Part model, mm, in its own coordinate system. A direction names the side the tool comes from. Coordinates: 2 decimals unless noted, no trailing zeros. Order: outer loops, then holes, each group sorted by start corner. A loop starts at its lowest first (then second) coordinate and runs counter-clockwise, first axis right, second up. Notation, with made-up numbers: M 62.5,63.25 L 120.5,63.25 A25 cw 120.5,96.25 Z; hole C -12,3.25 d4. An arc over 180 degrees is marked long. Answer in a Markdown table with one row per item. Add a question column.
from build123d import *

# Parameters (mm, degrees)
SKETCH1_W             = 24
SKETCH1_H             = 40
BOSS_EXTRUDE1_DEPTH   = 10
SKETCH2_R             = 4
BOSS_EXTRUDE2_DEPTH   = 10
SKETCH4_W             = 2
SKETCH4_H             = 15
CUT_EXTRUDE1_DEPTH    = 20
SKETCH5_R             = 2.4
CUT_EXTRUDE2_DEPTH    = 56
CHAMFER2_SIZE         = 2
CHAMFER3_SIZE2        = 2
CHAMFER3_SIZE         = 5.63516655
CHAMFER3_EDGE_2_SIZE2 = 5.63516655
CHAMFER3_EDGE_2_SIZE  = 2
CHAMFER3_EDGE_3_SIZE2 = 2
CHAMFER3_EDGE_3_SIZE  = 5.63516655
CHAMFER3_EDGE_4_SIZE2 = 5.63516655
CHAMFER3_EDGE_4_SIZE  = 2
FILLET2_R             = 3


with BuildPart() as part:
    # Sketch1 → Boss-Extrude1 (new body)
    with BuildSketch(Plane(origin=(0, 0, 0), x_dir=(1, 0, 0), z_dir=(0, 1, 0))):
        Rectangle(SKETCH1_W, SKETCH1_H)
    extrude(amount=BOSS_EXTRUDE1_DEPTH)

    # Sketch2 → Boss-Extrude2 (add)
    with BuildSketch(Plane.XZ):
        Polygon((-12, -20), (-12, 30), (-27, 30), (-27, -20), (-10, -30), (-10, -45), (10, -45), (10, -30), (27, -20), (27, 30), (12, 30), (12, -20), align=None)
        with Locations((0, -34)):
            Circle(SKETCH2_R, mode=Mode.SUBTRACT)
        with Locations((-19.5, 19)):
            Circle(SKETCH2_R, mode=Mode.SUBTRACT)
        with Locations((19.5, 19)):
            Circle(SKETCH2_R, mode=Mode.SUBTRACT)
    extrude(amount=-BOSS_EXTRUDE2_DEPTH)

    # Sketch4 → Cut-Extrude1 (cut)
    with BuildSketch(Plane(origin=(0, 10, 0), x_dir=(1, 0, 0), z_dir=(0, 1, 0))):
        with Locations((19.5, -30)):
            Rectangle(SKETCH4_W, SKETCH4_H)
        with Locations((-19.5, -30)):
            Rectangle(SKETCH4_W, SKETCH4_H)
        with Locations((0, 45)):
            Rectangle(SKETCH4_W, SKETCH4_H)
    extrude(amount=-CUT_EXTRUDE1_DEPTH, mode=Mode.SUBTRACT)

    # Sketch5 → Cut-Extrude2 (cut)
    with BuildSketch(Plane(origin=(27, 0, 0), x_dir=(0, 0, -1), z_dir=(1, 0, 0))):
        with Locations((-25.5, 5)):
            Circle(SKETCH5_R)
        with Locations((40.5, 5)):
            Circle(SKETCH5_R)
    extrude(amount=-CUT_EXTRUDE2_DEPTH, mode=Mode.SUBTRACT)

    # Chamfer2
    chamfer2_edges = [part.edges().sort_by_distance(p)[0] for p in [
        (-12, 5, 30),
        (12, 5, 30),
        (27, 5, 30),
        (10, 5, -45),
        (-10, 5, -45),
        (-27, 5, 30),
    ]]
    chamfer(chamfer2_edges, length=CHAMFER2_SIZE)

    # Chamfer3
    chamfer3_edges = [part.edges().sort_by_distance(p)[0] for p in [
        (27, 5, -20),
    ]]
    chamfer(chamfer3_edges, length=CHAMFER3_SIZE, length2=CHAMFER3_SIZE2)

    # Chamfer3 edge 2
    chamfer3_edge_2_edges = [part.edges().sort_by_distance(p)[0] for p in [
        (10, 5, -30),
    ]]
    chamfer(chamfer3_edge_2_edges, length=CHAMFER3_EDGE_2_SIZE, length2=CHAMFER3_EDGE_2_SIZE2)

    # Chamfer3 edge 3
    chamfer3_edge_3_edges = [part.edges().sort_by_distance(p)[0] for p in [
        (-10, 5, -30),
    ]]
    chamfer(chamfer3_edge_3_edges, length=CHAMFER3_EDGE_3_SIZE, length2=CHAMFER3_EDGE_3_SIZE2)

    # Chamfer3 edge 4
    chamfer3_edge_4_edges = [part.edges().sort_by_distance(p)[0] for p in [
        (-27, 5, -20),
    ]]
    chamfer(chamfer3_edge_4_edges, length=CHAMFER3_EDGE_4_SIZE, length2=CHAMFER3_EDGE_4_SIZE2)

    # Fillet2
    fillet2_edges = [part.edges().sort_by_distance(p)[0] for p in [
        (12, 5, 20),
        (-12, 5, 20),
    ]]
    fillet(fillet2_edges, radius=FILLET2_R)


solid = part.part
(1) Slice it at D-D (y = 5). State how many separate pieces and enclosed holes the cut face has, and give its area (3 significant figures).
(2) Slice it at C-C (z = -40.5). List the corners of the cut face in (x, y), and give its area (3 significant figures).
(3) Wall check: line 1 (X direction, y = 3.25, z = 19); line 2 (Z direction, x = -22.5, y = 7); line 3 (Z direction, x = 22, y = 4). Give the ranges that are in metal, low to high.
(4) Slice it at A-A (z = 19). List the corners of the cut face in (x, y).
(5) Drop flat-ended pins along their axis: P1, Ø2, axis at y = 2.5, z = -40, coming from the +X side; P2, Ø5, axis at x = -19.5, z = 19, coming from the +Y side; P3, Ø10, axis at x = 19, z = 10.5, coming from the -Y side; P4, Ø5.5, axis at y = 4, z = -43, coming from the -X side. Give the stop position or say it passes through.
(6) Slice it at B-B (x = -3). List the corners of the cut face in (y, z).
(7) 3-axis set-ups, long thin cutter, end or side, ignore diameter. For faces 5 (the flat face through (-10, 4.9, -37.6)), 6 (the flat face through (18.405, 4.93, -25.056)), 7 (the flat face through (-18.5, 5.1, 28.1)): which of +Z, -Z, +X, -X, +Y, -Y reach the whole face in a straight line?
(8) Pull direction Z, two halves, no side cores. Call faces 1 (the flat face through (23, 5, 30)), 2 (the cylindrical face through (-19.662, 4.93, 15.003)), 3 (the flat face through (10, 4.9, -37.7)), 4 (the cylindrical face through (-15.2, 5.72, 23.21)): pulls with the +Z half, pulls with the -Z half, needs draft (parallel to the pull), parting line crosses it, or undercut.
Computed:
| question | item | result |
|---|---|---|
| 1 | separate pieces | 7 |
| 1 | enclosed holes | 0 |
| 1 | area | 2,720 mm^2 |
| 2 | outline | M -10,0 L -1,0 L -1,2.6 L -10,2.6 Z; M -10,7.4 L -1,7.4 L -1,10 L -10,10 Z; M 1,0 L 10,0 L 10,2.6 L 1,2.6 Z; M 1,7.4 L 10,7.4 L 10,10 L 1,10 Z |
| 2 | area | 93.6 mm^2 |
| 3 | line 1 | x = -27 to -23.5, -15.5 to 15.5, 23.5 to 27 |
| 3 | line 2 | z = -22.65 to 16.35, 21.65 to 24.17, 26.83 to 30 |
| 3 | line 3 | z = -22.94 to 15.88, 22.12 to 23.32, 27.68 to 30 |
| 4 | outline | M -27,0 L -23.5,0 L -23.5,10 L -27,10 Z; M -15.5,0 L 15.5,0 L 15.5,10 L -15.5,10 Z; M 23.5,0 L 27,0 L 27,10 L 23.5,10 Z |
| 5 | P1 | stops at x = 10 |
| 5 | P2 | passes through |
| 5 | P3 | stops at y = 0 |
| 5 | P4 | stops at x = -10 |
| 6 | outline | M 0,-45 L 10,-45 L 10,-36.65 L 0,-36.65 Z; M 0,-31.35 L 10,-31.35 L 10,20 L 0,20 Z; hole C 5,-40.5 d4.8 |
| 7 | face 5 | -Z, -X, +Y, -Y |
| 7 | face 6 | -Z, +X, +Y, -Y |
| 7 | face 7 | +Z, +Y, -Y |
| 8 | face 1 | pulls with the +Z half |
| 8 | face 2 | undercut |
| 8 | face 3 | needs draft |
| 8 | face 4 | undercut |
